Part model, mm, in its own coordinate system. Face numbers are marked on the shaded views. Round coordinates to 2 decimals unless told otherwise and drop trailing zeros. Order: outer loops, then holes, each group sorted by start corner. A loop starts at its lowest first (then second) coordinate and runs counter-clockwise, first axis right, second up. Notation, with made-up numbers: M 58,-36 L 74,-36 A23 cw 74,-7 Z; hole C 39,42 d10. An arc over 180 degrees is marked long. Write each question's results on one line, items separated by ' | '. Start each with the question number.
1. Band-saw the part on B-B, the plane z = 17.5. List the corners of the cut face in (x, y).
2. Probe L1, parallel to Z at x = 0, y = 44; L2, parallel to X at y = 27.5, z = 0; L3, parallel to X at y = 56.5, z = 0. List the from-to ranges inside material, lowest first. Write a range as [from, to].
3. Band-saw the part on A-A, the plane x = 0. List the corners of the cut face in (y, z).
4. Two-plate mould, pull along Z, no slides. Class the marked faces 1, 2 and 3: +Z half, -Z half, draft (parallel to the pull), parting line (faces both ways), or undercut.
5. Band-saw the part on C-C, the plane y = 31. Give the number of separate pieces and of enclosed holes in the cut face, then the cut area to 3 significant figures.
6. Drop flat-ended pins along their axis: pin 1 Ø4 at (y, z) = (27.5, -21) entering from +X; pin 2 Ø6 at (x, y) = (59, 15) entering from +Z; pin 3 Ø2 at (y, z) = (13, -8.5) entering from -X. Give the stop position or say it passes through.
Autodesk Inventor part; units mm, degrees
ref_plane "工作平面2" through (38, 65.923, 0) normal (-0.997, -0.0769, 0) x (0.0769, -0.997, 0)
ref_plane "工作平面3" through (0, 0, 70) normal (0, 0, 1) x (1, 0, 0)
ref_plane "YZ Plane" through (0, 0, 0) normal (1, 0, 0) x (0, 1, 0)
sketch "草圖1" plane through (0, 0, 0) normal (0, 1, 0) x (-1, 0, 0)
  circle A0 centre (0, 0) radius 40
  dimension "d0" = 80
extrude "擠出1" add sketch "草圖1" along normal blind 80
shell "薄殼3" thickness 2 removed faces 1 at (12.1058, 80, -2.3153)
sketch "草圖6" plane through (0, 0, 0) normal (0, 0, 1) x (1, 0, 0)
  line L0 (40, 0) -> (40, 80)
  arc A0 (38, 14.077) -> (38, 65.923) centre (40, 40) ccw
  line L1 (-40, 0) -> (40, 0)
  line L2 (38, 2) -> (38, 80) construction
  point P0 (0, 0)
  dimension "d23" = 52
  dimension "d24" = 40
ref_plane "工作平面2" through (38, 65.923, 0) normal (-0.997, -0.0769, 0) x (0.0769, -0.997, 0)
sketch "草圖7" plane through (38, 65.923, 0) normal (-0.997, -0.0769, 0) x (0.0769, -0.997, 0)
  ellipse E0 centre (0, 0) end of major axis (0, -6) minor radius 4
  point P0 (62.8046, 0)
  dimension "d25" = 4
  dimension "d26" = 6
sweep "掃掠3" add profiles "草圖7" path "草圖6" path curves A0
fillet "圓角5" radius 2 2 edges at (39.5474, 66.0021, 6) (39.5474, 13.9979, 6)
ref_plane "工作平面3" through (0, 0, 70) normal (0, 0, 1) x (1, 0, 0)
sketch "草圖11" plane through (0, 0, 70) normal (0, 0, 1) x (1, 0, 0)
  line L0 (-18.4453, 56.0809) -> (19.5727, 56.0809)
  line L1 (19.5727, 56.0809) -> (19.5727, 18.0629)
  line L2 (19.5727, 18.0629) -> (-18.4453, 18.0629)
  line L3 (-18.4453, 18.0629) -> (-18.4453, 56.0809)
  point P0 (0, 0)
decal "印花2"
properties part number "練習二"
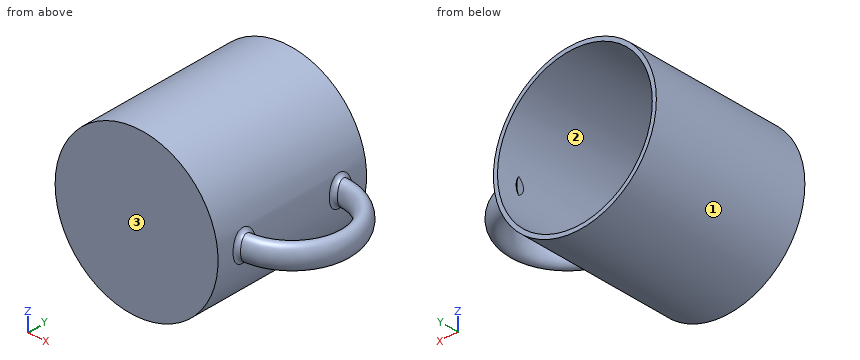
Solution:
1) outline: M -35.97,0 L 35.97,0 L 35.97,80 L 33.73,80 L 33.73,2 L -33.73,2 L -33.73,80 L -35.97,80 Z
2) L1: [-40, -38], [38, 40] | L2: [-40, -38], [38, 40], [58.1, 67.27] | L3: [-40, -38], [38, 40], [54.55, 65.05]
3) outline: M 0,-40 L 80,-40 L 80,-38 L 2,-38 L 2,38 L 80,38 L 80,40 L 0,40 Z
4) face 1: parting line | face 2: undercut | face 3: draft
5) separate pieces: 2 | enclosed holes: 1 | area: 571 mm^2
6) pin 1: x = 35.2 | pin 2: z = 4.8 | pin 3: x = -39.29
